Can you work these out from the model? Positions are in its coordinate system, mm. Give positions to 0.01 mm unless a question says otherwise; leave off trailing zeros. Write each loop counter-clockwise with the first axis right and the second up, starting at its lowest first coordinate (ties: lowest second). Pieces come first, ordered by that corner, then holes.
1. Suppose I cut it at A-A (y = -76.2). Please give me the cut outline in (x, z) (1 decimal).
2. Suppose I cut it at D-D (y = -135). Please give me the cut outline in (x, z) (3 decimals), and give its area (3 significant figures).
3. I'm going to push flat-ended pins straight in: pin 1 (1 mm diameter, centred on y = -67.5, z = 2, fed in from +X); pin 2 (1 mm diameter, centred on y = -33.5, z = 2, fed in from -X); pin 3 (1.6 mm diameter, centred on x = -2, z = 1.5, fed in from +Y). Where does each tip first touch, or does it pass through?
4. Thinking about a two-plate mould opening in Y: for faces 1 (the flat face through (113, -88, 3.175)), 2 (the cylindrical face through (118.7, -78.02, 1.57)), which applies, pulls with the +Y half, pulls with the -Y half, needs draft (parallel to the pull), parting line crosses it, or undercut?
5. Suppose I cut it at B-B (x = 114.3). Please give me the cut outline in (y, z) (1 decimal).
6. If I drill on probe 1 along Y at (x, z) = (114.3, 1); probe 2 along X at (y, z) = (-115, 2.2); probe 3 along Y at (x, z) = (111, 2.6), over which ranges is the centre line in solid material (lowest first)?
```python
from build123d import *

# Parameters (mm, degrees)
F0_R     = 4.7625
F0_W     = 3.175
F0_H     = 6.35
F1_DEPTH = 3.175


# Not quite as in the source:
# - a length typed as a fraction of an inch, garbled in the dataset ("3 / 203.2 mm" for 3/8 in), is restored


with BuildPart() as f1:
    # F0 (on Top) → F1 (new body)
    with BuildSketch(Plane.XY):
        Polygon((228.6, 0), (0, 0), (0, -6.35), (0, -152.4), (0, -158.75), (0, -171.45), (0, -177.8), (228.6, -177.8), (228.6, -171.45), (228.6, -158.75), (228.6, -152.4), (228.6, -6.35), align=None)
        with Locations((114.3, -76.2)):
            Circle(F0_R, mode=Mode.SUBTRACT)
        with Locations((-1.5875, -155.575)):
            Rectangle(F0_W, F0_H)
        with Locations((-1.5875, -174.625)):
            Rectangle(F0_W, F0_H)
        with Locations((-1.5875, -3.175)):
            Rectangle(F0_W, F0_H)
        with Locations((230.1875, -3.175)):
            Rectangle(F0_W, F0_H)
        with Locations((230.1875, -155.575)):
            Rectangle(F0_W, F0_H)
        with Locations((230.1875, -174.625)):
            Rectangle(F0_W, F0_H)
    extrude(amount=F1_DEPTH)


solid = f1.part
```
Checks:
1. outline: (0, 0) - (109.5, 0) - (109.5, 3.2) - (0, 3.2) - close; (119.1, 0) - (228.6, 0) - (228.6, 3.2) - (119.1, 3.2) - close
2. outline: (0, 0) - (228.6, 0) - (228.6, 3.175) - (0, 3.175) - close
2. area: 726 mm2
3. pin 1: stops at x = 228.6
3. pin 2: stops at x = 0
3. pin 3: stops at y = 0
4. face 1: needs draft
4. face 2: undercut
5. outline: (-177.8, 0) - (-81, 0) - (-81, 3.2) - (-177.8, 3.2) - close; (-71.4, 0) - (0, 0) - (0, 3.2) - (-71.4, 3.2) - close
6. probe 1: y = -177.8 to -80.96, -71.44 to 0
6. probe 2: x = 0 to 228.6
6. probe 3: y = -177.8 to -79.63, -72.77 to 0
